```python
from build123d import *

# Parameters (mm, degrees)
SKETCH_1_W      = 92
SKETCH_1_H      = 88
SKETCH_1_R      = 1.6
SKETCH_1_R_2    = 1.5
EXTRUDE_1_DEPTH = 3


with BuildPart() as part:
    # 草图1 → 凸台-拉伸1 (new body)
    with BuildSketch(Plane.XY):
        with Locations((46, 44)):
            Rectangle(SKETCH_1_W, SKETCH_1_H)
        with Locations((5, 8)):
            Circle(SKETCH_1_R, mode=Mode.SUBTRACT)
        with Locations(Location((5, 80, 0), (0, 0, 180))):
            Circle(SKETCH_1_R, mode=Mode.SUBTRACT)
        with Locations(Location((87, 8, 0), (0, 0, 180))):
            Circle(SKETCH_1_R, mode=Mode.SUBTRACT)
        with Locations((87, 80)):
            Circle(SKETCH_1_R, mode=Mode.SUBTRACT)
        with Locations((46, 81)):
            Circle(SKETCH_1_R_2, mode=Mode.SUBTRACT)
        with Locations((77.5, 44)):
            Circle(SKETCH_1_R_2, mode=Mode.SUBTRACT)
        with Locations(Location((46, 7, 0), (0, 0, 180))):
            Circle(SKETCH_1_R_2, mode=Mode.SUBTRACT)
        with Locations(Location((14.5, 44, 0), (0, 0, 180))):
            Circle(SKETCH_1_R_2, mode=Mode.SUBTRACT)
    extrude(amount=EXTRUDE_1_DEPTH)


solid = part.part
```
Build history of the part. All positions in model axes, mm. Give positions to 0.01 mm unless a question says otherwise; leave off trailing zeros. Loops run counter-clockwise (first coordinate to the right, second up) from the corner with the lowest first, then second, coordinate; pieces in that order, holes last.
Item 1: Drill centre lines: line 1 (Y direction, x = 5, z = 1.4); line 2 (Y direction, x = 77.5, z = 2); line 3 (X direction, y = 81, z = 2.2). Where is each one in solid material? Low to high.
Answers follow:
line 1: y = 0 to 6.4, 9.6 to 78.4, 81.6 to 88
line 2: y = 0 to 42.5, 45.5 to 88
line 3: x = 0 to 3.75, 6.25 to 44.5, 47.5 to 85.75, 88.25 to 92
Item 2: Slice it at A-A, the plane x = 5. List the corners of the cut face in (y, z).
Answers follow:
outline: (0, 0) - (6.4, 0) - (6.4, 3) - (0, 3) - close; (9.6, 0) - (78.4, 0) - (78.4, 3) - (9.6, 3) - close; (81.6, 0) - (88, 0) - (88, 3) - (81.6, 3) - close
Item 3: Pull direction Y, two halves, no side cores. Call faces 1 (the face through (85.4, 80.07, 1.48)), 2 (the face through (45, 88, 1)), 3 (the face through (45, 0, 1)), 4 (the face through (45, 45, 0)): released by +Y, released by -Y, zero draft, split by the parting line, or undercut.
Answers follow:
face 1: undercut
face 2: released by +Y
face 3: released by -Y
face 4: zero draft
Item 4: Slice it at B-B, the plane y = 44. List the corners of the cut face in (x, z).
Answers follow:
outline: (0, 0) - (13, 0) - (13, 3) - (0, 3) - close; (16, 0) - (76, 0) - (76, 3) - (16, 3) - close; (79, 0) - (92, 0) - (92, 3) - (79, 3) - close
Item 5: Flat gauge pin, fed straight in: pin 1 (5 mm diameter, centred on x = 46, y = 81, fed in from -Z). Where does the tip first touch, or does it go through?
Answers follow:
pin 1: stops at z = 0
Item 6: Slice it at C-C, the plane x = 77.5. List the corners of the cut face in (y, z), and give its area (3 significant figures).
Answers follow:
outline: (0, 0) - (42.5, 0) - (42.5, 3) - (0, 3) - close; (45.5, 0) - (88, 0) - (88, 3) - (45.5, 3) - close
area: 255 mm2
